from build123d import *

# Parameters (mm, degrees)
SKETCH_W        = 8.1
SKETCH_H        = 36
PAD_DEPTH       = 4.05
SKETCH001_R     = 2.85
POCKET_DEPTH    = 20
SKETCH002_R     = 0.655
POCKET001_DEPTH = 16
SKETCH003_W     = 12.15
SKETCH003_H     = 10
POCKET002_DEPTH = 4.05
FILLET_R        = 0.5


with BuildPart() as part:
    # Sketch → Pad (new body, symmetric)
    with BuildSketch(Plane.XY):
        with Locations((0, 18)):
            Rectangle(SKETCH_W, SKETCH_H)
    extrude(amount=PAD_DEPTH, both=True)

    # Sketch001 → Pocket (cut)
    with BuildSketch(Plane.XZ):
        Circle(SKETCH001_R)
    extrude(amount=-POCKET_DEPTH, mode=Mode.SUBTRACT)

    # Sketch002 (on DatumPlane) → Pocket001 (cut)
    with BuildSketch(Plane(origin=(0, 36, 0), x_dir=(-1, 0, 0), z_dir=(0, 1, 0))):
        Circle(SKETCH002_R)
    extrude(amount=-POCKET001_DEPTH, mode=Mode.SUBTRACT)

    # Sketch003 (on DatumPlane) → Pocket002 (cut)
    with BuildSketch(Plane.XY.offset(4.05)):
        with Locations((0, 25)):
            Rectangle(SKETCH003_W, SKETCH003_H)
    extrude(amount=-POCKET002_DEPTH, mode=Mode.SUBTRACT)

    # Fillet
    fillet_edges = [part.edges().sort_by_distance(p)[0] for p in [
        (4.05, 36, 0),
        (0, 36, 4.05),
        (-4.05, 36, 0),
        (4.05, 33, 4.05),
        (-4.05, 33, 4.05),
        (-4.05, 10, 4.05),
        (4.05, 0, 0),
        (0, 0, 4.05),
        (-4.05, 0, 0),
        (4.05, 10, 4.05),
        (4.05, 20, 2.025),
        (4.05, 25, 0),
        (0, 20, 4.05),
        (-4.05, 20, 2.025),
        (-4.05, 25, 0),
        (-4.05, 30, 2.025),
        (0, 30, 4.05),
    ]]
    fillet(fillet_edges, radius=FILLET_R)


solid = part.part
Work out the finished part from the listing and answer in its coordinate system (mm). A direction names the side the tool comes from. Give positions to 0.01 mm unless a question says otherwise; leave off trailing zeros. Write each loop counter-clockwise with the first axis right and the second up, starting at its lowest first coordinate (ties: lowest second). Pieces come first, ordered by that corner, then holes. Notation, with made-up numbers: M -16,-37.75 L 21,-37.75 A8 ccw 21,-30.75 Z; hole C 29,-21 d5. An arc over 180 degrees is marked long. Answer as CSV lines item,"result".
Q1. A cutting plane is placed at A-A on y = 14.5. Write down the section's boundary in (x, z).
A:
outline,"M -4.05,-4.05 L 4.05,-4.05 L 4.05,3.55 A0.5 ccw 3.55,4.05 L -3.55,4.05 A0.5 ccw -4.05,3.55 Z; hole C 0,0 d5.7"
Q2. Given P1, Ø0.9, axis at x = 0, z = -1.5, coming from the -Y side; P2, Ø1, axis at x = 0, z = 0, coming from the -Y side; P3, Ø2, axis at x = 2, y = 27.5, coming from the +Z side, each flat-ended and moving along its own axis, determine where each tip first touches the part or whether it passes through.
A:
P1,"stops at y = 20"
P2,"passes through"
P3,"stops at z = 0"
Q3. Find the intervals of material crossed by probe 1 along Z at (x, y) = (0, 32.5) (3 decimals); probe 2 along Y at (x, z) = (1.5, 2.75), in increasing order. Write a range as [from, to].
A:
probe 1,"z = [-4.05, -0.655], [0.655, 4.05]"
probe 2,"y = [0, 20], [30, 36]"
Q4. A cutting plane is placed at D-D on x = 2. Write down the section's boundary in (y, z).
A:
outline,"M 0,-4.05 L 36,-4.05 L 36,3.55 A0.5 ccw 35.5,4.05 L 30.5,4.05 A0.5 ccw 30,3.55 L 30,0 L 20,0 L 20,-2.03 L 0,-2.03 Z; M 0,2.03 L 20,2.03 L 20,3.55 A0.5 ccw 19.5,4.05 L 0.5,4.05 A0.5 ccw 0,3.55 Z"
Q5. A cutting plane is placed at C-C on z = 2. Write down the section's boundary in (x, y).
A:
outline,"M -4.05,0.5 A0.5 ccw -3.55,0 L -2.03,0 L -2.03,20 L -3.55,20 A0.5 ccw -4.05,19.5 Z; M -4.05,30.5 A0.5 ccw -3.55,30 L 4.05,30 L 4.05,35.5 A0.5 ccw 3.55,36 L -3.55,36 A0.5 ccw -4.05,35.5 Z; M 2.03,0 L 3.55,0 A0.5 ccw 4.05,0.5 L 4.05,19.5 A0.5 ccw 3.55,20 L 2.03,20 Z"
Q6. A tool of negligible diameter and unlimited length cuts with its end or side. For faces 4 (the flat face through (-4.05, 18, 0)), 5 (the flat face through (2, 25, 0)), 6 (the flat face through (0, 20, -1)), from which of +Z, -Z, +X, -X, +Y, -Y can it reach the whole face along a straight path? Write none if from no direction.
A:
face 4,"+Z, -Z, -X, +Y, -Y"
face 5,"+Z, +X, -X"
face 6,"-Y"
Q7. A cutting plane is placed at B-B on x = 0. Write down the section's boundary in (y, z) (3 decimals), plus the area to 3 significant figures.
A:
outline,"M 0,-4.05 L 36,-4.05 L 36,-0.655 L 20,-0.655 L 20,-2.85 L 0,-2.85 Z; M 0,2.85 L 20,2.85 L 20,3.55 A0.5 ccw 19.5,4.05 L 0.5,4.05 A0.5 ccw 0,3.55 Z; M 30,0.655 L 36,0.655 L 36,3.55 A0.5 ccw 35.5,4.05 L 30.5,4.05 A0.5 ccw 30,3.55 Z"
area,"122 mm²"
Q8. The mould has two halves that part along X. Classify faces 1 (the cylindrical face through (-2.262, 9.86, -1.734)), 2 (the flat face through (0, 33, 4.05)), 3 (the flat face through (4.05, 18, 0)): +X half, -X half, draft (parallel to the pull), parting line (faces both ways), or undercut.
A:
face 1,"undercut"
face 2,"draft"
face 3,"+X half"
